Could you check a few things on this drawing? It's one solid part, dimensions in mm from its lowest x, y, z. A direction names the side the tool comes from. Coordinates: 2 decimals unless noted, no trailing zeros. Loops run counter-clockwise (first coordinate to the right, second up) from the corner with the lowest first, then second, coordinate; pieces in that order, holes last. Notation, with made-up numbers: (-1, -17.5) -> (40, -17.5) arc R19 ccw to (40, -4.5) -> close; hole circle Ø8 at (76, 65.5). An arc over 180 degrees is marked (long way). One line per question, with ' | ' between items. Start each with the question number.
(1) I'm going to push flat-ended pins straight in: pin 1 Ø4 at (y, z) = (2.5, 33) entering from +X (1 decimal); pin 2 Ø8.5 at (x, z) = (12, 16) entering from +Y; pin 3 Ø2 at (y, z) = (2, 8) entering from +X. Where does each tip first touch, or does it pass through?
(2) Which directions (+Z, -Z, +X, -X, +Y, -Y) give clear straight access to the entire face, cutting with the end or side of a thin tool? Please do the marked faces 5 and 6.
(3) If I drill on line 1 along X through (y, z) = (4, 20.5); line 2 along Y through (x, z) = (6.5, 12.5); line 3 along Z through (x, y) = (12, 2.25) (1 decimal), over which ranges is the centre line in solid material (lowest first)?
(4) Suppose I cut it at A-A (y = 9.25). Please give me the cut outline in (x, z) (1 decimal).
(5) If we mould it in two halves opening along X, with no side actions, what happens to the marked faces 1, 2, 3 and 4? For each: pulls with the +X half, pulls with the -X half, needs draft (parallel to the pull), parting line crosses it, or undercut.
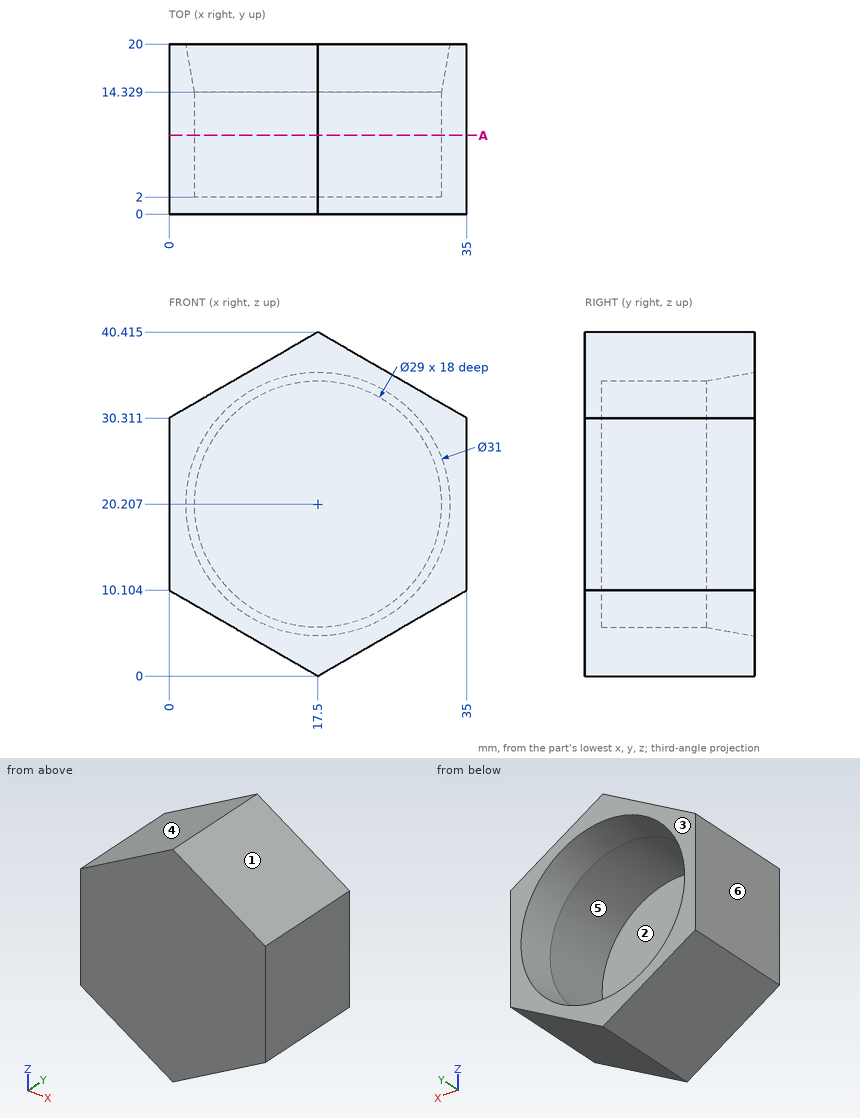
Checks:
1) pin 1: stops at x = 33.8 | pin 2: stops at y = 2 | pin 3: stops at x = 33.09
2) face 5: +Y | face 6: +Z, -Z, -X, +Y, -Y
3) line 1: x = 0 to 3, 32 to 35 | line 2: y = 0 to 2 | line 3: z = 3.2 to 6.8, 33.6 to 37.2
4) outline: (0, 10.1) -> (17.5, 0) -> (35, 10.1) -> (35, 30.3) -> (17.5, 40.4) -> (0, 30.3) -> close; hole circle Ø29 at (17.5, 20.2)
5) face 1: pulls with the +X half | face 2: undercut | face 3: needs draft | face 4: pulls with the -X half
